Input: part model. Units: mm. Frame: model coordinates. Face numbers are marked on the shaded views. A direction names the side the tool comes from. Round coordinates to 2 decimals unless told otherwise and drop trailing zeros. Loops run counter-clockwise (first coordinate to the right, second up) from the corner with the lowest first, then second, coordinate; pieces in that order, holes last. Notation, with made-up numbers: (-36, 35.25) - (-13, 35.25) arc R16 cw to (-13, 63.25) - close; hole circle Ø8 at (67.25, 50.5). An arc over 180 degrees is marked (long way). One line per question, with ' | ' between items. Start each with the question number.
Item 1: Section A-A, the plane z = 0. Return loops of the section in (x, y), plus the area to 3 significant figures.
Item 2: Set-up query: the marked faces 1, 2 and 3. Return all of +Z, -Z, +X, -X, +Y, -Y with unobstructed straight access to the full face (end or side cutting, diameter ignored); none if empty.
Item 3: First-contact query: pin 1 (1.5 mm diameter, centred on x = -10.5, y = 5, fed in from -Z); pin 2 (2.5 mm diameter, centred on x = 10.5, y = 5, fed in from -Z); pin 3 (6 mm diameter, centred on x = -9.5, z = 0, fed in from +Y). Flat tips, straight axial feed; report the tip coordinate or a pass-through.
Item 4: Section D-D, the plane y = 1.5. Return loops of the section in (x, z), plus the area to 3 significant figures.
Item 5: Section C-C, the plane x = 9.5. Return loops of the section in (y, z), plus the area to 3 significant figures.
Item 6: Draft query along Z for the marked faces 4, 5 and 6. Return one class per face: pulls with the +Z half, pulls with the -Z half, needs draft (parallel to the pull), parting line crosses it, or undercut.
Item 7: Material intervals for line 1 along Z through (x, y) = (0, 3); line 2 along X through (y, z) = (0.75, 0); line 3 along Z through (x, y) = (0, 0.5), sorted ascending.
Item 8: Section B-B, the plane y = 5.5. Return loops of the section in (x, z), plus the area to 3 significant figures.
```python
from build123d import *

# Parameters (mm, degrees)
SKETCH1_R         = 15
SKETCH1_R_2       = 4.7
BASE_DEPTH        = 2
TRIANGLES_DEPTH   = 5
FILLET1_R         = 1.25
WHEEL_HOLES_REACH = 4
SKETCH3_R         = 1.8
SKETCH4_R         = 1.25
HORN_HOLES_DEPTH  = 8


with BuildPart() as part:
    # Sketch1 → Base (new body)
    with BuildSketch(Plane(origin=(0, 0, 0), x_dir=(1, 0, 0), z_dir=(0, 1, 0))):
        Circle(SKETCH1_R)
        Circle(SKETCH1_R_2, mode=Mode.SUBTRACT)
    extrude(amount=BASE_DEPTH)

    # Sketch2 → Triangles (add)
    with BuildSketch(Plane(origin=(0, 2, 0), x_dir=(1, 0, 0), z_dir=(0, 1, 0))):
        with BuildLine():
            Line((6.028500388, 3.557693505), (14.571422537, 3.560006353))
            ThreePointArc((14.571422537, 3.560006353), (12.959336441, 7.553515672), (10.279001399, 10.924382373))
            Line((10.279001399, 10.924382373), (6.028500388, 3.557693505))
        make_face()
        with BuildLine():
            Line((-0.066802761, 6.999681235), (4.202655329, 14.399225263))
            ThreePointArc((4.202655329, 14.399225263), (-0.061868239, 14.99987241), (-4.321291956, 14.364067524))
            Line((-4.321291956, 14.364067524), (-0.066802761, 6.999681235))
        make_face()
        with BuildLine():
            Line((6.095303148, -3.44198773), (10.368767208, -10.83921891))
            ThreePointArc((10.368767208, -10.83921891), (13.02120468, -7.446356739), (14.600293355, -3.439685151))
            Line((14.600293355, -3.439685151), (6.095303148, -3.44198773))
        make_face()
        with BuildLine():
            Line((0.066802761, -6.999681235), (-4.202655329, -14.399225263))
            ThreePointArc((-4.202655329, -14.399225263), (0.061868239, -14.99987241), (4.321291956, -14.364067524))
            Line((4.321291956, -14.364067524), (0.066802761, -6.999681235))
        make_face()
        with BuildLine():
            Line((-6.028500388, -3.557693505), (-14.571422537, -3.560006353))
            ThreePointArc((-14.571422537, -3.560006353), (-12.959336441, -7.553515672), (-10.279001399, -10.924382373))
            Line((-10.279001399, -10.924382373), (-6.028500388, -3.557693505))
        make_face()
        with BuildLine():
            Line((-6.095303148, 3.44198773), (-10.368767208, 10.83921891))
            ThreePointArc((-10.368767208, 10.83921891), (-13.02120468, 7.446356739), (-14.600293355, 3.439685151))
            Line((-14.600293355, 3.439685151), (-6.095303148, 3.44198773))
        make_face()
    extrude(amount=TRIANGLES_DEPTH)

    # Fillet1
    fillet1_edges = [part.edges().sort_by_distance(p)[0] for p in [
        (6.095303148, 4.5, 3.44198773),
        (0.066802761, 4.5, 6.999681235),
        (-6.028500388, 4.5, 3.557693505),
        (-6.095303148, 4.5, -3.44198773),
        (6.028500388, 4.5, -3.557693505),
        (-0.066802761, 4.5, -6.999681235),
    ]]
    fillet(fillet1_edges, radius=FILLET1_R)

    # Sketch3 → Wheel Holes (cut, up to next)
    with BuildSketch(Plane(origin=(0, 2, 0), x_dir=(1, 0, 0), z_dir=(0, 1, 0)), mode=Mode.PRIVATE) as wheel_holes_sk1:
        with Locations((-9.5, 0)):
            Circle(SKETCH3_R)
    wheel_holes_tool1 = extrude(wheel_holes_sk1.sketch, amount=-WHEEL_HOLES_REACH, mode=Mode.PRIVATE) & part.part
    add(wheel_holes_tool1.solids().sort_by_distance((-9.5, 2, 0))[0], mode=Mode.SUBTRACT)
    # Sketch3 → Wheel Holes (cut, up to next)
    with BuildSketch(Plane(origin=(0, 2, 0), x_dir=(1, 0, 0), z_dir=(0, 1, 0)), mode=Mode.PRIVATE) as wheel_holes_sk2:
        with Locations((9.5, 0)):
            Circle(SKETCH3_R)
    wheel_holes_tool2 = extrude(wheel_holes_sk2.sketch, amount=-WHEEL_HOLES_REACH, mode=Mode.PRIVATE) & part.part
    add(wheel_holes_tool2.solids().sort_by_distance((9.5, 2, 0))[0], mode=Mode.SUBTRACT)

    # Sketch4 → Horn Holes (cut, through all)
    with BuildSketch(Plane(origin=(0, 7, 0), x_dir=(1, 0, 0), z_dir=(0, 1, 0))):
        with Locations((0, 13.25)):
            Circle(SKETCH4_R)
        with Locations((0, -13.25)):
            Circle(SKETCH4_R)
    extrude(amount=-HORN_HOLES_DEPTH, mode=Mode.SUBTRACT)


solid = part.part
```
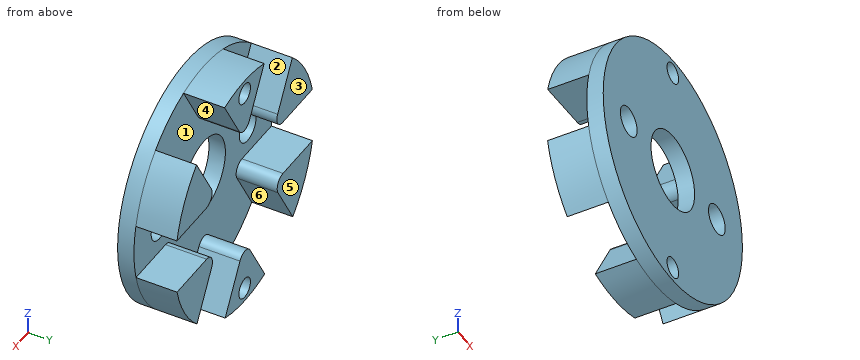
Return value:
1) outline: (-15, 0) - (-11.3, 0) - (-11.3, 2) - (-15, 2) - close; (-7.7, 0) - (-4.7, 0) - (-4.7, 2) - (-7.7, 2) - close; (4.7, 0) - (7.7, 0) - (7.7, 2) - (4.7, 2) - close; (11.3, 0) - (15, 0) - (15, 2) - (11.3, 2) - close | area: 26.8 mm2
2) face 1: +Y | face 2: +Z, +Y | face 3: +Z, -Z, +X, -X, +Y
3) pin 1: z = -10.84 | pin 2: z = -10.92 | pin 3: y = 2
4) outline: circle Ø30 at (0, 0); hole circle Ø3.6 at (-9.5, 0); hole circle Ø9.4 at (0, 0); hole circle Ø2.5 at (0, -13.25); hole circle Ø2.5 at (0, 13.25); hole circle Ø3.6 at (9.5, 0) | area: 607 mm2
5) outline: (0, -11.61) - (2, -11.61) - (2, -9.57) - (7, -9.57) - (7, -3.56) - (2, -3.56) - (2, -1.8) - (0, -1.8) - close; (0, 1.8) - (2, 1.8) - (2, 3.44) - (7, 3.44) - (7, 9.34) - (2, 9.34) - (2, 11.61) - (0, 11.61) - close | area: 98.8 mm2
6) face 4: undercut | face 5: needs draft | face 6: pulls with the -Z half
7) line 1: -15 to -14.5, -12 to -8.25, 8.25 to 12, 14.5 to 15 | line 2: -15 to -11.3, -7.7 to -4.7, 4.7 to 7.7, 11.3 to 15 | line 3: -15 to -14.5, -12 to -4.7, 4.7 to 12, 14.5 to 15
8) outline: (-14.6, -3.44) arc R15 ccw to (-10.37, -10.84) - (-7.18, -5.32) arc R1.25 ccw to (-8.26, -3.44) - close; (-14.57, 3.56) - (-8.19, 3.56) arc R1.25 ccw to (-7.11, 5.43) - (-10.28, 10.92) arc R15 ccw to start; (-4.32, -14.36) arc R15 ccw to (4.2, -14.4) - (1.02, -8.87) arc R1.25 ccw to (-1.15, -8.87) - close; (-4.2, 14.4) - (-1.02, 8.87) arc R1.25 ccw to (1.15, 8.87) - (4.32, 14.36) arc R15 ccw to start; (7.11, -5.43) - (10.28, -10.92) arc R15 ccw to (14.57, -3.56) - (8.19, -3.56) arc R1.25 ccw to start; (7.18, 5.32) arc R1.25 ccw to (8.26, 3.44) - (14.6, 3.44) arc R15 ccw to (10.37, 10.84) - close; hole circle Ø2.5 at (0, -13.25); hole circle Ø2.5 at (0, 13.25) | area: 194 mm2
